Verification items for the finished model (mm, model axes). Give positions to 0.01 mm unless a question says otherwise; leave off trailing zeros. Order: outer loops, then holes, each group sorted by start corner. A loop starts at its lowest first (then second) coordinate and runs counter-clockwise, first axis right, second up. Notation, with made-up numbers: M 88.25,68.25 L 113.25,68.25 A12 cw 113.25,72.25 Z; hole C 84.25,-9 d2. An arc over 180 degrees is marked long. Answer as a JSON object with one key per item and string values.
Autodesk Inventor part; units mm, degrees
ref_plane "YZ Plane" through (0, 0, 0) normal (1, 0, 0) x (0, 1, 0)
ref_plane "XZ Plane" through (0, 0, 0) normal (0, 1, 0) x (-1, 0, 0)
ref_plane "XY Plane" through (0, 0, 0) normal (0, 0, 1) x (1, 0, 0)
sketch "Эскиз1" plane through (0, 0, 0) normal (0, 0, 1) x (1, 0, 0)
  line L0 (-18.939, -15) -> (19.061, -15)
  line L1 (19.061, -15) -> (19.061, 10)
  line L2 (19.061, 10) -> (-18.939, 10)
  line L3 (-18.939, 10) -> (-18.939, -15)
  circle A0 centre (-14.939, 5) radius 1.6
  circle A1 centre (-14.939, -9) radius 1.6
  circle A2 centre (15.061, 5) radius 1.6
  circle A3 centre (15.061, -9) radius 1.6
  point P0 (0, 0)
  dimension "d0" = 38
  dimension "d5" = 3.2
  dimension "d7" = 14
  dimension "d16" = 3.2
  dimension "d17" = 3.2
  dimension "d18" = 3.2
  dimension "d19" = 5
  dimension "d20" = 14
  dimension "d21" = 6
  dimension "d22" = 6
  dimension "d23" = 4
  dimension "d25" = 4
  dimension "d26" = 4
extrude "Выдавливание1" add sketch "Эскиз1" along normal blind 2
chamfer "Фаска1" distance 4 angle 45 4 edges at (19.061, 10, 1) (-18.939, 10, 1) (19.061, -15, 1) (-18.939, -15, 1)
properties part number "стена_простая"
Q1. Material ranges on L1, parallel to X at y = -7.75, z = 1.7; L2, parallel to X at y = -8, z = 0.6; L3, parallel to Y at x = 14, z = 0.9, recorded low to high.
Resolved:
{"L1": "x = -18.94 to -15.94, -13.94 to 14.06, 16.06 to 19.06", "L2": "x = -18.94 to -16.19, -13.69 to 13.81, 16.31 to 19.06", "L3": "y = -15 to -10.2, -7.8 to 3.8, 6.2 to 10"}
Q2. Release check for a two-part mould opening along X. For faces 1 (the face through (-16.91, -13.03, 1.01)), 2 (the face through (16.587, 4.519, 0.986)), 3 (the face through (19.061, -3, 1)), 4 (the face through (-13.46, -8.39, 0.99)) record: +X half, -X half, draft (parallel to the pull), parting line (faces both ways), or undercut.
Resolved:
{"face 1": "-X half", "face 2": "undercut", "face 3": "+X half", "face 4": "undercut"}
Q3. Section check C-C on y = 8. Record the cut outline in (x, z).
Resolved:
{"outline": "M -16.94,0 L 17.06,0 L 17.06,2 L -16.94,2 Z"}
Q4. Section check A-A on y = -9. Record the cut outline in (x, z), then the cut area to 3 significant figures.
Resolved:
{"outline": "M -18.94,0 L -16.54,0 L -16.54,2 L -18.94,2 Z; M -13.34,0 L 13.46,0 L 13.46,2 L -13.34,2 Z; M 16.66,0 L 19.06,0 L 19.06,2 L 16.66,2 Z", "area": "63.2 mm²"}
Q5. Section check B-B on z = 1.1. Record the cut outline in (x, y).
Resolved:
{"outline": "M -18.94,-11 L -14.94,-15 L 15.06,-15 L 19.06,-11 L 19.06,6 L 15.06,10 L -14.94,10 L -18.94,6 Z; hole C -14.94,-9 d3.2; hole C -14.94,5 d3.2; hole C 15.06,-9 d3.2; hole C 15.06,5 d3.2"}
